Autodesk Inventor part; units mm, degrees
ref_plane "YZ Plane" through (0, 0, 0) normal (1, 0, 0) x (0, 1, 0)
ref_plane "XZ Plane" through (0, 0, 0) normal (0, 1, 0) x (-1, 0, 0)
ref_plane "XY Plane" through (0, 0, 0) normal (0, 0, 1) x (1, 0, 0)
sketch "Sketch1" plane through (0, 0, 0) normal (0, 0, 1) x (1, 0, 0)
  circle A0 centre (0, 0) radius 98.425
  circle A1 centre (0, 0) radius 142.875
  dimension "d0" = 196.85
  dimension "d1" = 44.45
extrude "Extrusion1" add sketch "Sketch1" along normal blind 6.35
sketch "Sketch2" plane through (0, 0, 6.35) normal (0, 0, 1) x (1, 0, 0)
  circle A0 centre (0, 120.269) radius 2.5797
  line L0 (0, 120.269) -> (0, 0) construction
  line L1 (0, 0) -> (23.4633, 117.9581) construction
  line L2 (0, 0) -> (51.0308, 123.1993) construction
  line L3 (0, 0) -> (63.5017, 95.037) construction
  circle A1 centre (23.4633, 117.9581) radius 4.445
  circle A2 centre (-85.043, 85.043) radius 2.5797
  circle A3 centre (-66.8179, 100) radius 4.445
  circle A4 centre (-120.269, 0) radius 2.5797
  circle A5 centre (-117.9581, 23.4633) radius 4.445
  circle A6 centre (-85.043, -85.043) radius 2.5797
  circle A7 centre (-100, -66.8179) radius 4.445
  circle A8 centre (0, -120.269) radius 2.5797
  circle A9 centre (-23.4633, -117.9581) radius 4.445
  circle A10 centre (85.043, -85.043) radius 2.5797
  circle A11 centre (66.8179, -100) radius 4.445
  circle A12 centre (120.269, 0) radius 2.5797
  circle A13 centre (117.9581, -23.4633) radius 4.445
  circle A14 centre (85.043, 85.043) radius 2.5797
  circle A15 centre (100, 66.8179) radius 4.445
  circle A16 centre (51.0308, 123.1993) radius 2.5797
  circle A17 centre (46.1708, 111.4661) radius 2.5797
  circle A18 centre (41.3107, 99.7328) radius 2.5797
  circle A19 centre (59.9738, 89.7571) radius 6.35
  line L4 (59.9738, 89.7571) -> (0, 0)
  circle A20 centre (-21.06, 105.8758) radius 6.35
  circle A21 centre (-89.7571, 59.9738) radius 6.35
  circle A22 centre (-105.8758, -21.06) radius 6.35
  circle A23 centre (-59.9738, -89.7571) radius 6.35
  circle A24 centre (21.06, -105.8758) radius 6.35
  circle A25 centre (89.7571, -59.9738) radius 6.35
  circle A26 centre (105.8758, 21.06) radius 6.35
  circle A27 centre (-41.3107, 99.7328) radius 2.5797
  circle A28 centre (-46.1708, 111.4661) radius 2.5797
  circle A29 centre (-51.0308, 123.1993) radius 2.5797
  circle A30 centre (-99.7328, 41.3107) radius 2.5797
  circle A31 centre (-111.4661, 46.1708) radius 2.5797
  circle A32 centre (-123.1993, 51.0308) radius 2.5797
  circle A33 centre (-99.7328, -41.3107) radius 2.5797
  circle A34 centre (-111.4661, -46.1708) radius 2.5797
  circle A35 centre (-123.1993, -51.0308) radius 2.5797
  circle A36 centre (-41.3107, -99.7328) radius 2.5797
  circle A37 centre (-46.1708, -111.4661) radius 2.5797
  circle A38 centre (-51.0308, -123.1993) radius 2.5797
  circle A39 centre (41.3107, -99.7328) radius 2.5797
  circle A40 centre (46.1708, -111.4661) radius 2.5797
  circle A41 centre (51.0308, -123.1993) radius 2.5797
  circle A42 centre (99.7328, -41.3107) radius 2.5797
  circle A43 centre (111.4661, -46.1708) radius 2.5797
  circle A44 centre (123.1993, -51.0308) radius 2.5797
  circle A45 centre (99.7328, 41.3107) radius 2.5797
  circle A46 centre (111.4661, 46.1708) radius 2.5797
  circle A47 centre (123.1993, 51.0308) radius 2.5797
  circle A48 centre (0, 133.35) radius 2.5797
  circle A49 centre (-94.2927, 94.2927) radius 2.5797
  circle A50 centre (-133.35, 0) radius 2.5797
  circle A51 centre (-94.2927, -94.2927) radius 2.5797
  circle A52 centre (0, -133.35) radius 2.5797
  circle A53 centre (94.2927, -94.2927) radius 2.5797
  circle A54 centre (133.35, 0) radius 2.5797
  circle A55 centre (94.2927, 94.2927) radius 2.5797
  dimension "d4" = 5.1594
  dimension "d5" = 120.269
  dimension "d6" = 11.25
  dimension "d7" = 22.5
  dimension "d8" = 33.75
  dimension "d9" = 8.89
  dimension "d12" = 360
  dimension "d14" = 133.35
  dimension "d17" = 12.7
  dimension "d22" = 114.3
  dimension "d36" = 12.7
  dimension "d37" = 107.95
  dimension "d38" = 33.75
  dimension "d41" = 360
  dimension "d45" = 360
  dimension "d47" = 133.35
  dimension "d50" = 360
extrude "Extrusion2" cut sketch "Sketch2" against normal blind 6.35 contours A0 | A1 | A2 | A3 | A4 | A5 | A6 | A7 | A8 | A9 | A10 | A11 | A12 | A13 | A14 | A15 | A16 | A17 | A18 | A19 | A20 | A21 | A22 | A23 | A24 | A25 | A26 | A27 | A28 | A29 | A30 | A31 | A32 | A33 | A34 | A35 | A36 | A37 | A38 | A39 | A40 | A41 | A42 | A43 | A44 | A45 | A46 | A47
equation "\"d38\" = d8"
properties part number "IntakeCCenterWheelInterposer"
Here's how the part is built. I have some questions about the finished solid (model axes, mm). Round coordinates to 2 decimals unless told otherwise and drop trailing zeros. Order: outer loops, then holes, each group sorted by start corner. A loop starts at its lowest first (then second) coordinate and runs counter-clockwise, first axis right, second up. Notation, with made-up numbers: M 19,18 L 34,18 A27 ccw 34,56 Z; hole C 14,62.25 d1. An arc over 180 degrees is marked long. Answer as CSV lines item,"result".
Item 1: Imagine slicing it at B-B on y = -76.5. List the corners of the cut face in (x, z) for me.
From the geometry:
outline,"M -120.67,0 L -61.93,0 L -61.93,6.35 L -120.67,6.35 Z; M 61.93,0 L 120.67,0 L 120.67,6.35 L 61.93,6.35 Z"
Item 2: Imagine slicing it at C-C on z = 4. Give the number of separate pieces and of enclosed holes in the cut face, and give its area (3 significant figures).
From the geometry:
separate pieces,"1"
enclosed holes,"49"
area,"31,500 mm2"
Item 3: Imagine slicing it at A-A on x = 7.5. List the corners of the cut face in (y, z) for me.
From the geometry:
outline,"M -142.68,0 L -98.14,0 L -98.14,6.35 L -142.68,6.35 Z; M 98.14,0 L 142.68,0 L 142.68,6.35 L 98.14,6.35 Z"
Item 4: We'd pull the mould along X, two halves only. Please class faces 1 (the flat face through (-34, -93, 6.35)), 2 (the cylindrical face through (93.88, -29.56, 3.13)): +X half, -X half, draft (parallel to the pull), parting line (faces both ways), or undercut.
From the geometry:
face 1,"draft"
face 2,"undercut"
Item 5: For pin 1 (4.5 mm diameter, centred on x = 0, y = 120.269, fed in from +Z); pin 2 (3 mm diameter, centred on x = -110, z = 5, fed in from +Y), each with a flat end and sliding along its axis, tell me the tip position at first contact or that it passes through.
From the geometry:
pin 1,"through"
pin 2,"y = 92.96"
Item 6: Please list where these lines run through material, in increasing order: L1, parallel to Y at x = 61.5, z = 1.25; L2, parallel to Y at x = -113, z = 5.75; L3, parallel to X at y = 65, z = 2.5. Write a range as [from, to].
From the geometry:
L1,"[-128.96, -76.85], [76.85, 83.59], [95.92, 128.96]"
L2,"[-87.43, -48.24], [-44.1, 44.1], [48.24, 87.43]"
L3,"[-127.23, -93.64], [-85.88, -73.91], [73.91, 95.94], [104.06, 127.23]"
